```python
from build123d import *

# Parameters (mm, degrees)
F1_DEPTH = 78.3291
F2_R     = 7.7099954694
F3_DEPTH = 68.99092
F5_DEPTH = 11.99651
F6_R     = 2.7645751725
F7_DEPTH = 66.7321124816


with BuildPart() as f1:
    # F0 (on Front) → F1 (new body)
    with BuildSketch(Plane.XZ):
        Polygon((-72.8069469333, 0), (0, 0), (-40.571808815, 52.7989305556), (-72.8069469333, 52.7989305556), align=None)
    extrude(amount=F1_DEPTH)

    # F2 (on face) → F3 (cut)
    with BuildSketch(Plane(origin=(-72.8069469333, 0, 0), x_dir=(0, -1, 0), z_dir=(-1, 0, 0))):
        with Locations((37.1266901493, 27.6962798089)):
            Circle(F2_R)
    extrude(amount=-F3_DEPTH, mode=Mode.SUBTRACT)

    # F4 (on face) → F5 (join)
    with BuildSketch(Plane(origin=(0, 0, 0), x_dir=(-1, 0, 0), z_dir=(0, 1, 0))):
        Polygon((0, 0), (40.571808815, 52.7989305556), (72.8069469333, 52.7989305556), (72.8069469333, 63.7013316154), (37.4180935323, 63.7013316154), (-11.033478193, 0), align=None)
    extrude(amount=-F5_DEPTH)

    # F6 (on face) → F7 (cut, through all)
    with BuildSketch(Plane(origin=(6.9897594118, 0, 5.3164481949), x_dir=(0, 1, 0), z_dir=(0.7959300347, 0, 0.6053886188))):
        with Locations((-5.998255, 33.3373744617)):
            Circle(F6_R)
    extrude(amount=-F7_DEPTH, mode=Mode.SUBTRACT)


solid = f1.part
```
Can you work these out from the model? Positions are in its coordinate system, mm. A direction names the side the tool comes from. Round coordinates to 2 decimals unless told otherwise and drop trailing zeros. Loops run counter-clockwise (first coordinate to the right, second up) from the corner with the lowest first, then second, coordinate; pieces in that order, holes last.
Item 1: Please list where these lines run through material, in increasing order: L1, parallel to Z at x = -41, y = -61.5; L2, parallel to Z at x = -25.5, y = -5.5; L3, parallel to Y at x = -35, z = 29.
Item 2: Will these pins go through, and if not, where does the flat tip stop? pin 1 Ø5 at (y, z) = (-64.5, 51.5) entering from +X; pin 2 Ø10 at (y, z) = (-16.5, 8) entering from +X; pin 3 Ø3 at (y, z) = (-46, 18.5) entering from +X.
Item 3: Suppose I cut it at A-A, the plane z = 25. State how many separate pieces and enclosed holes the cut face has, then the cut area to 3 significant figures.
Item 4: Suppose I cut it at D-D, the plane z = 42. Write out the boundary of the cut face in (x, y).
Item 5: Suppose I cut it at B-B, the plane x = -5. Write out the boundary of the cut face in (y, z), then the cut area to 4 significant figures.
Item 6: Suppose I cut it at C-C, the plane y = -54. Write out the boundary of the cut face in (x, z).
Item 7: Which directions (+Z, -Z, +X, -X, +Y, -Y) give clear straight access to the entire face, cutting with the end or side of a thin tool? Please do faces 1 (the flat face through (-20, -52.07, 26.03)), 2 (the flat face through (-72.807, -29.9, 31.4)), 3 (the flat face through (-56, -45, 52.799)).
Item 8: If we mould it in two halves opening along Y, with no side actions, what happens to faces 4 (the cylindrical face through (-36.923, -6.358, 17.245)), 5 (the flat face through (-45, -78.329, 21)), 6 (the flat face through (-55, -6, 63.701)), 7 (the cylindrical face through (-44.41, -35.46, 20.17))? For each: +Y half, -Y half, draft (parallel to the pull), parting line (faces both ways), or undercut.
Reported:
1. L1: z = 0 to 52.8
1. L2: z = 0 to 19.07, 25.91 to 48.03
1. L3: y = -78.33 to -44.73, -29.53 to 0
2. pin 1: stops at x = -37.65
2. pin 2: stops at x = 6.6
2. pin 3: stops at x = -13.06
3. separate pieces: 2
3. enclosed holes: 1
3. area: 3,520 mm2
4. outline: (-72.81, -78.33) - (-32.27, -78.33) - (-32.27, -12) - (-20.91, -12) - (-20.91, 0) - (-72.81, 0) - close
5. outline: (-78.33, 0) - (0, 0) - (0, 21.08) - (-12, 21.08) - (-12, 6.51) - (-78.33, 6.51) - close
5. area: 684.5 mm2
6. outline: (-72.81, 0) - (0, 0) - (-40.57, 52.8) - (-72.81, 52.8) - close
7. face 1: +Z, +X, -Y
7. face 2: +Z, -Z, -X, +Y, -Y
7. face 3: +Z, +X, -X, -Y
8. face 4: undercut
8. face 5: -Y half
8. face 6: draft
8. face 7: undercut
